from build123d import *

# Parameters (mm, degrees)
ESQUISSE1_R                         = 16.5
BOSS_EXTRU_1_DEPTH                  = 25
BOSS_EXTRU_4_DEPTH                  = 12
BOSS_EXTRU_4_DEPTH_BACK             = 4
ESQUISSE9_R                         = 11.25
ESQUISSE10_R                        = 4.8
ENL_V_MAT_EXTRU_3_DEPTH             = 13
ESQUISSE11_R                        = 4
ENL_V_MAT_EXTRU_4_DEPTH             = 3.5
ENL_V_MAT_EXTRU_5_REACH             = 40.66
ENL_V_MAT_EXTRU_5_END_RADIUS        = 4.8
ESQUISSE12_R                        = 2
ESQUISSE13_R                        = 12.5
BOSS_EXTRU_5_DEPTH                  = 70
ESQUISSE15_R                        = 8
BOSS_EXTRU_6_DEPTH                  = 1.2
ESQUISSE2_R                         = 4.75
ENL_V_MAT_EXTRU_6_DEPTH             = 40
ENL_V_MAT_EXTRU_6_DIRECTION_2_REACH = 102.546


with BuildPart() as part:
    # Esquisse1 → Boss.-Extru.1 (new body)
    with BuildSketch(Plane(origin=(0, 0, 0), x_dir=(1, 0, 0), z_dir=(0, 1, 0))):
        with Locations(Location((0, 0, 0), (0, 0, 270))):
            Circle(ESQUISSE1_R)
    extrude(amount=BOSS_EXTRU_1_DEPTH)

    # Esquisse9 → Boss.-Extru.4 (add, two sides: drawn at the far end of the back side and taken through both)
    with BuildSketch(Plane(origin=(16.5, 0, 0), x_dir=(0, 0, -1), z_dir=(1, 0, 0)).offset(-BOSS_EXTRU_4_DEPTH_BACK)):
        with Locations((0, 12.5)):
            Circle(ESQUISSE9_R)
    extrude(amount=BOSS_EXTRU_4_DEPTH + BOSS_EXTRU_4_DEPTH_BACK)

    # Esquisse10 → Enlèv. mat.-Extru.3 (cut)
    with BuildSketch(Plane(origin=(28.5, 0, 0), x_dir=(0, 0, -1), z_dir=(1, 0, 0))):
        with Locations((0, 12.5)):
            Circle(ESQUISSE10_R)
    extrude(amount=-ENL_V_MAT_EXTRU_3_DEPTH, mode=Mode.SUBTRACT)

    # Esquisse11 → Enlèv. mat.-Extru.4 (cut)
    with BuildSketch(Plane(origin=(0, 1.25, 0), x_dir=(1, 0, 0), z_dir=(0, 1, 0))):
        with Locations(Location((22, 0, 0), (0, 0, 90))):
            Circle(ESQUISSE11_R)
    enl_v_mat_extru_4 = extrude(amount=ENL_V_MAT_EXTRU_4_DEPTH, mode=Mode.SUBTRACT)

    # Enlèv. mat.-Extru.5: up to this cylinder (the profile starts outside it)
    enl_v_mat_extru_5_end = Plane(origin=(22, 12.5, 0), z_dir=(1, 0, 0)) * Cylinder(ENL_V_MAT_EXTRU_5_END_RADIUS, 91.92, mode=Mode.PRIVATE)
    # Esquisse12 → Enlèv. mat.-Extru.5 (cut, up to the surface)
    with BuildSketch(Plane.XZ.offset(-4.75), mode=Mode.PRIVATE) as enl_v_mat_extru_5_sk1:
        with Locations(Location((22, 0, 0), (0, 0, 270))):
            Circle(ESQUISSE12_R)
    enl_v_mat_extru_5_tool1 = extrude(enl_v_mat_extru_5_sk1.sketch, amount=-ENL_V_MAT_EXTRU_5_REACH, mode=Mode.PRIVATE) - enl_v_mat_extru_5_end
    enl_v_mat_extru_5 = enl_v_mat_extru_5_tool1.solids().sort_by_distance((22, 4.75, 0))[0]
    add(enl_v_mat_extru_5, mode=Mode.SUBTRACT)

    # Symétrie1: Enlèv. mat.-Extru.4, Enlèv. mat.-Extru.5 across plane
    add(enl_v_mat_extru_4.mirror(Plane.XY), mode=Mode.SUBTRACT)
    add(enl_v_mat_extru_5.mirror(Plane.XY), mode=Mode.SUBTRACT)

    # Symétrie1 at the second plane: Enlèv. mat.-Extru.4, Enlèv. mat.-Extru.5 across plane
    add(enl_v_mat_extru_4.mirror(Plane.ZX.offset(12.5)), mode=Mode.SUBTRACT)
    add(enl_v_mat_extru_5.mirror(Plane.ZX.offset(12.5)), mode=Mode.SUBTRACT)

    # Esquisse13 → Boss.-Extru.5 (add)
    with BuildSketch(Plane(origin=(0, 25, 0), x_dir=(1, 0, 0), z_dir=(0, 1, 0))):
        with Locations(Location((0, 0, 0), (0, 0, 270))):
            Circle(ESQUISSE13_R)
    extrude(amount=BOSS_EXTRU_5_DEPTH)

    # Esquisse15 → Boss.-Extru.6 (add)
    with BuildSketch(Plane.XZ):
        with Locations(Location((0, 0, 0), (0, 0, 270))):
            Circle(ESQUISSE15_R)
    extrude(amount=BOSS_EXTRU_6_DEPTH)

    # Esquisse2 → Enlèv. mat.-Extru.6 (cut)
    with BuildSketch(Plane.XZ):
        with Locations(Location((0, 0, 0), (0, 0, 270))):
            Circle(ESQUISSE2_R)
    extrude(amount=-ENL_V_MAT_EXTRU_6_DEPTH, mode=Mode.SUBTRACT)

    # Esquisse2 → Enlèv. mat.-Extru.6 direction 2 (cut, up to next)
    with BuildSketch(Plane.XZ, mode=Mode.PRIVATE) as enl_v_mat_extru_6_direction_2_sk1:
        with Locations(Location((0, 0, 0), (0, 0, 270))):
            Circle(ESQUISSE2_R)
    enl_v_mat_extru_6_direction_2_tool1 = extrude(enl_v_mat_extru_6_direction_2_sk1.sketch, amount=ENL_V_MAT_EXTRU_6_DIRECTION_2_REACH, mode=Mode.PRIVATE) & part.part
    add(enl_v_mat_extru_6_direction_2_tool1.solids().sort_by_distance((0, 0, 0))[0], mode=Mode.SUBTRACT)


solid = part.part
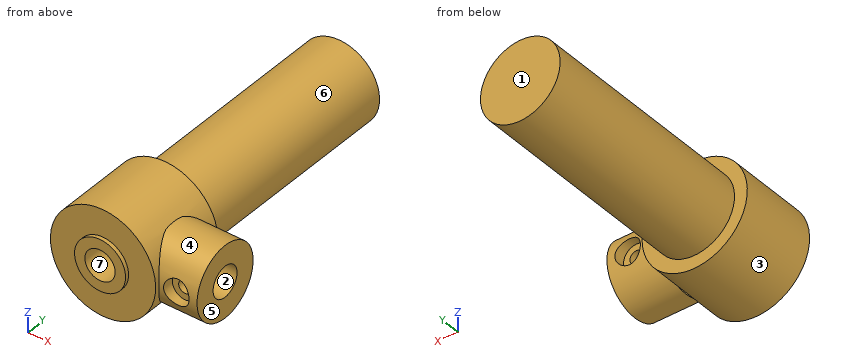
Input: part model. Units: mm. Frame: model coordinates. Face numbers are marked on the shaded views. A direction names the side the tool comes from. Give positions to 0.01 mm unless a question says otherwise; leave off trailing zeros. Order: outer loops, then holes, each group sorted by start corner. A loop starts at its lowest first (then second) coordinate and runs counter-clockwise, first axis right, second up.
Q1. Contact query for flat-ended pins moving along their axis: pin 1 Ø8 at (y, z) = (62.5, 4.5) entering from +X; pin 2 Ø4 at (x, z) = (21.5, 1) entering from -Y; pin 3 Ø4.5 at (x, z) = (22, 0) entering from +Y; pin 4 Ø11 at (y, z) = (12.5, 0) entering from +X. Output: stop coordinate, or through.
Checked values:
pin 1: stops at x = 12.49
pin 2: stops at y = 4.75
pin 3: stops at y = 20.25
pin 4: stops at x = 28.5
Q2. Ray query, probe 1 along X at (y, z) = (19, 0); probe 2 along X at (y, z) = (2, 0); probe 3 along X at (y, z) = (27.5, 0). Return the intervals inside material, ascending.
Checked values:
probe 1: x = -16.5 to -4.75, 4.75 to 20, 24 to 28.5
probe 2: x = -16.5 to -4.75, 4.75 to 18, 26 to 28.5
probe 3: x = -12.5 to -4.75, 4.75 to 12.5
Q3. Set-up query: the marked faces 4, 5, 6 and 7. Return all of +Z, -Z, +X, -X, +Y, -Y with unobstructed straight access to the full face (end or side cutting, diameter ignored); none if empty.
Checked values:
face 4: +X
face 5: +Z, -Z, +X, +Y, -Y
face 6: +Y
face 7: -Y
Q4. Section C-C on z = 0. State how many separate pieces and enclosed holes the cut face has, and give its area (3 significant figures).
Checked values:
separate pieces: 3
enclosed holes: 0
area: 2,270 mm2
Q5. Draft query along Z for the marked faces 1, 2 and 3. Return one class per face: +Z half, -Z half, draft (parallel to the pull), parting line (faces both ways), or undercut.
Checked values:
face 1: draft
face 2: undercut
face 3: parting line
Q6. Section D-D on x = 0. Output: boundary loops of the cut face in (y, z).
Checked values:
outline: (-1.2, -8) - (0, -8) - (0, -16.5) - (25, -16.5) - (25, -12.5) - (95, -12.5) - (95, 12.5) - (25, 12.5) - (25, 16.5) - (0, 16.5) - (0, 8) - (-1.2, 8) - (-1.2, 4.75) - (40, 4.75) - (40, -4.75) - (-1.2, -4.75) - close
Q7. Section B-B on x = 22. Output: boundary loops of the cut face in (y, z).
Checked values:
outline: (1.99, -4) arc R11.25 ccw to (23.01, -4) - (20.25, -4) - (20.25, -2) - (16.86, -2) arc R4.8 cw to (8.14, -2) - (4.75, -2) - (4.75, -4) - close; (1.99, 4) - (4.75, 4) - (4.75, 2) - (8.14, 2) arc R4.8 cw to (16.86, 2) - (20.25, 2) - (20.25, 4) - (23.01, 4) arc R11.25 ccw to start
Q8. Section A-A on y = 12.5. Output: boundary loops of the cut face in (x, z).
Checked values:
outline: (12.5, -11.25) - (28.5, -11.25) - (28.5, -4.8) - (15.5, -4.8) - (15.5, 4.8) - (28.5, 4.8) - (28.5, 11.25) - (12.5, 11.25) - (12.5, 10.77) arc R16.5 ccw (long way) to (12.5, -10.77) - close; hole circle Ø9.5 at (0, 0)
